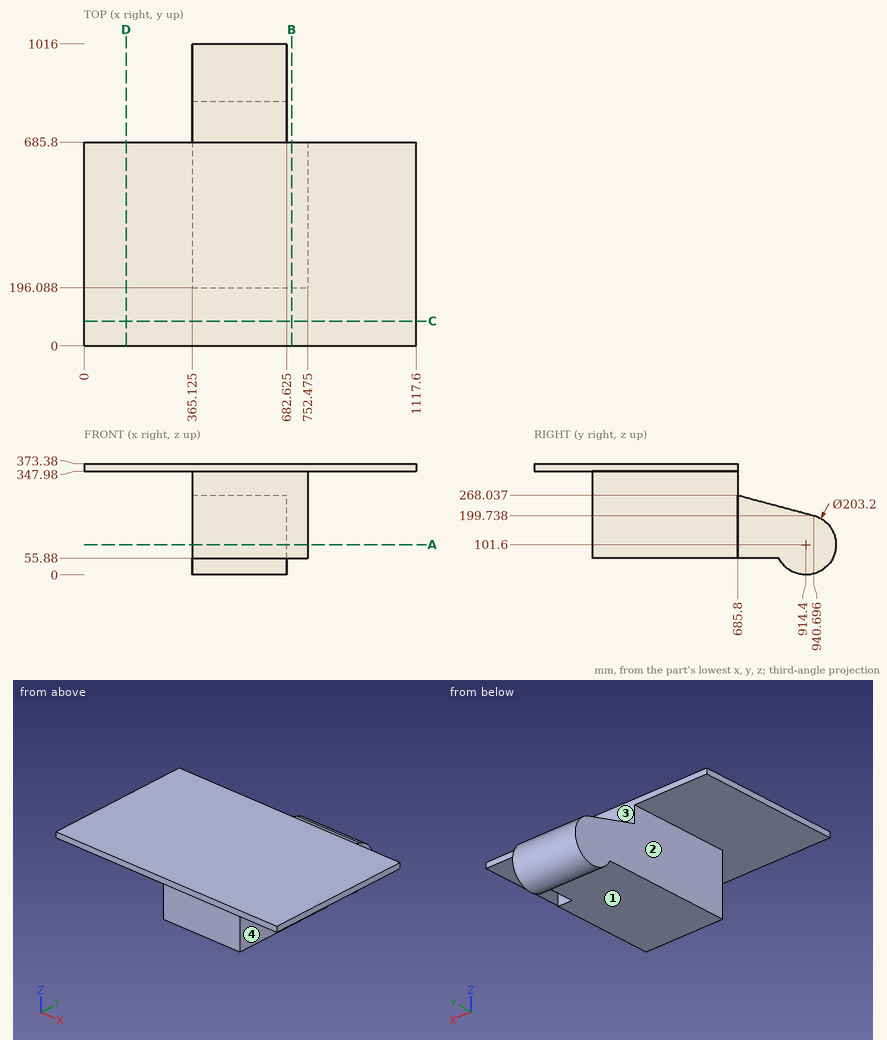
Input: dimensioned drawing with shaded views. Units: mm. Origin: part minimum x, y, z. A direction names the side the tool comes from. Give positions to 0.01 mm unless a question says otherwise; leave off trailing zeros. Write each loop counter-clockwise with the first axis right and the second up, starting at its lowest first coordinate (ties: lowest second). Pieces come first, ordered by that corner, then holes. Notation, with made-up numbers: (-2, 16) - (36, 16) arc R19 ccw to (36, 23) - close; hole circle Ø3 at (47.25, -38.5). An arc over 180 degrees is marked (long way). Write item = value, one per line. Start each with the question number.
1) Reachability of the marked faces 1, 2, 3 and 4 from +Z, -Z, +X, -X, +Y, -Y: full face, straight path, thin tool, end or side. Return the list, or none.
2) Material intervals for L1, parallel to X at y = 678, z = 321 (3 decimals); L2, parallel to Y at x = 511.5, z = 281; L3, parallel to Z at x = 231.5, y = 514.5, sorted ascending. Write a range as [from, to].
3) Cut plane B-B (x = 699). Return loops of the section in (y, z).
4) Cut plane C-C (y = 83). Return loops of the section in (x, z), and give its area (3 significant figures).
5) Cut plane D-D (x = 141.5). Return loops of the section in (y, z).
6) Cut plane A-A (z = 101.6). Return loops of the section in (x, y) (3 decimals).
7) Pin query (flat end, axial travel): pin 1 (5 mm diameter, centred on y = 272.5, z = 323, fed in from +X) (3 decimals); pin 2 (6 mm diameter, centred on x = 508, y = 753.5, fed in from -Z); pin 3 (1.5 mm diameter, centred on x = 241.5, y = 482.5, fed in from -Z). Return the tip coordinate at first contact, or that it passes through.
Answers follow:
q1.face_1 = -Z, +X, -X, -Y
q1.face_2 = -Z, -X, +Y, -Y
q1.face_3 = +Z, +X, +Y
q1.face_4 = -Z, +X, +Y, -Y
q2.L1 = [365.125, 752.475]
q2.L2 = [196.09, 685.8]
q2.L3 = [347.98, 373.38]
q3.outline = (0, 347.98) - (196.09, 347.98) - (196.09, 55.88) - (685.8, 55.88) - (685.8, 373.38) - (0, 373.38) - close
q4.outline = (0, 347.98) - (1117.6, 347.98) - (1117.6, 373.38) - (0, 373.38) - close
q4.area = 28,400 mm^2
q5.outline = (0, 347.98) - (685.8, 347.98) - (685.8, 373.38) - (0, 373.38) - close
q6.outline = (365.125, 196.088) - (752.475, 196.088) - (752.475, 685.8) - (682.625, 685.8) - (682.625, 1016) - (365.125, 1016) - close
q7.pin_1 = 752.475
q7.pin_2 = 55.88
q7.pin_3 = 347.98
